For this review, take the finished solid that the model builds, in its own axes (mm). Face numbers are marked on the shaded views. Give positions to 0.01 mm unless a question says otherwise; leave off trailing zeros. Loops run counter-clockwise (first coordinate to the right, second up) from the corner with the lowest first, then second, coordinate; pieces in that order, holes last. Notation, with made-up numbers: (11.25, 38.5) - (57.25, 38.5) arc R22 ccw to (57.25, 71.5) - close; hole circle Ø11 at (49, 85.25). An arc over 180 degrees is marked (long way). Put each result on its own line as item: value.
from build123d import *

# Parameters (mm, degrees)
SKETCH_1_R      = 1.5
SKETCH_1_R_2    = 5
EXTRUDE_1_DEPTH = 3


with BuildPart() as part:
    # 草图1 → 凸台-拉伸1 (new body)
    with BuildSketch(Plane(origin=(0, 0, 0), x_dir=(-1, 0, 0), z_dir=(0, 1, 0))):
        with BuildLine():
            Line((-3.031088913, 21.75), (-20.351596989, -8.25))
            ThreePointArc((-20.351596989, -8.25), (-20.351596989, -11.75), (-17.320508076, -13.5))
            Line((-17.320508076, -13.5), (17.320508076, -13.5))
            ThreePointArc((17.320508076, -13.5), (20.351596989, -11.75), (20.351596989, -8.25))
            Line((20.351596989, -8.25), (3.031088913, 21.75))
            ThreePointArc((3.031088913, 21.75), (0, 23.5), (-3.031088913, 21.75))
        make_face()
        with Locations((0, 20)):
            Circle(SKETCH_1_R, mode=Mode.SUBTRACT)
        with Locations((17.320508076, -10)):
            Circle(SKETCH_1_R, mode=Mode.SUBTRACT)
        with Locations((-17.320508076, -10)):
            Circle(SKETCH_1_R, mode=Mode.SUBTRACT)
        with Locations((-5.196152423, 3)):
            Circle(SKETCH_1_R, mode=Mode.SUBTRACT)
        Circle(SKETCH_1_R, mode=Mode.SUBTRACT)
        with Locations((0, 10.5)):
            Circle(SKETCH_1_R_2, mode=Mode.SUBTRACT)
        with Locations((9.09326674, -5.25)):
            Circle(SKETCH_1_R_2, mode=Mode.SUBTRACT)
        with Locations((-9.09326674, -5.25)):
            Circle(SKETCH_1_R_2, mode=Mode.SUBTRACT)
        with Locations((0, -6)):
            Circle(SKETCH_1_R, mode=Mode.SUBTRACT)
        with Locations((5.196152423, 3)):
            Circle(SKETCH_1_R, mode=Mode.SUBTRACT)
    extrude(amount=EXTRUDE_1_DEPTH)


solid = part.part
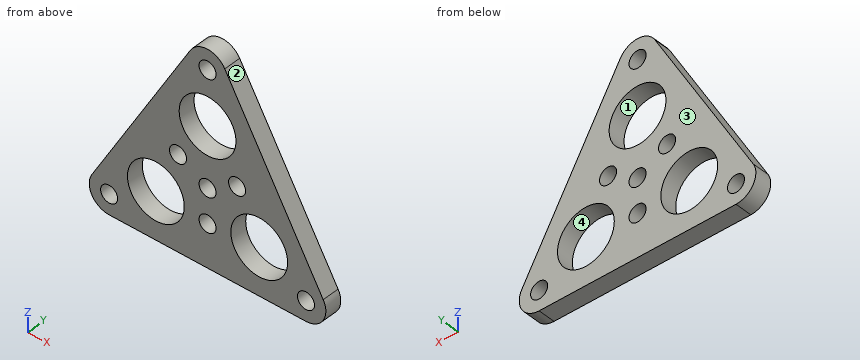
1) Take a section at B-B on z = -5.25. State the section outline as (x, y) points, and give its area (3 significant figures).
Geometry check:
outline: (-18.62, 0) - (-14.09, 0) - (-14.09, 3) - (-18.62, 3) - close; (-4.09, 0) - (-1.3, 0) - (-1.3, 3) - (-4.09, 3) - close; (1.3, 0) - (4.09, 0) - (4.09, 3) - (1.3, 3) - close; (14.09, 0) - (18.62, 0) - (18.62, 3) - (14.09, 3) - close
area: 43.9 mm²
2) Insertion check: pin 1 Ø1 at (x, y) = (9.5, 2.5) entering from +Z; pin 2 Ø1.5 at (x, y) = (-16, 0.5) entering from +Z. Each pin has a flat end and moves straight along its axis. Give the tip position at first contact, or say it passes through.
Geometry check:
pin 1: stops at z = 11.41
pin 2: stops at z = 0.59
3) Draft analysis for pull direction Z (two halves, no side actions). For the marked faces 1, 2, 3 and 4, state which applies: pulls with the +Z half, pulls with the -Z half, needs draft (parallel to the pull), parting line crosses it, or undercut.
Geometry check:
face 1: undercut
face 2: pulls with the +Z half
face 3: needs draft
face 4: undercut
4) Take a section at D-D on x = -8.5. State the section outline as (y, z) points.
Geometry check:
outline: (0, -13.5) - (3, -13.5) - (3, -10.21) - (0, -10.21) - close; (0, -0.29) - (3, -0.29) - (3, 12.28) - (0, 12.28) - close
5) Take a section at C-C on y = 0.95. State how many separate pieces and enclosed holes the cut face has, and give its area (3 significant figures).
Geometry check:
separate pieces: 1
enclosed holes: 10
area: 637 mm²
6) Take a section at A-A on x = 0. State the section outline as (y, z) points, and give its area (3 significant figures).
Geometry check:
outline: (0, -13.5) - (3, -13.5) - (3, -7.5) - (0, -7.5) - close; (0, -4.5) - (3, -4.5) - (3, -1.5) - (0, -1.5) - close; (0, 1.5) - (3, 1.5) - (3, 5.5) - (0, 5.5) - close; (0, 15.5) - (3, 15.5) - (3, 18.5) - (0, 18.5) - close; (0, 21.5) - (3, 21.5) - (3, 23.5) - (0, 23.5) - close
area: 54.0 mm²
7) Wall thickness on line 1 (Z direction, x = -0.5, y = 2.75); line 2 (Z direction, x = 0, y = 1.55); line 3 (X direction, y = 0.85, z = -5): over which ranges is each line inside the solid? List them lowest first.
Geometry check:
line 1: z = -13.5 to -7.41, -4.59 to -1.41, 1.41 to 5.53, 15.47 to 18.59, 21.41 to 23.46
line 2: z = -13.5 to -7.5, -4.5 to -1.5, 1.5 to 5.5, 15.5 to 18.5, 21.5 to 23.5
line 3: x = -18.48 to -14.09, -4.1 to -1.12, 1.12 to 4.1, 14.09 to 18.48
